Work out the finished part from the listing and answer in its coordinate system (mm). A direction names the side the tool comes from. Round coordinates to 2 decimals unless told otherwise and drop trailing zeros. Loops run counter-clockwise (first coordinate to the right, second up) from the corner with the lowest first, then second, coordinate; pieces in that order, holes last. Notation, with made-up numbers: (48.5, 79) -> (63.5, 79) arc R25 cw to (63.5, 97) -> close; hole circle Ø8 at (-4, 88.25). An arc over 180 degrees is marked (long way). Use CSV: the item, a comma, the result in double quotes. Start each with the question number.
from build123d import *

# Parameters (mm, degrees)
BOSS_EXTRUDE1_DEPTH = 76.2
CUT_EXTRUDE1_DEPTH  = 105.116765701
SKETCH3_R           = 1.5875
CUT_EXTRUDE2_DEPTH  = 105.116765701


with BuildPart() as part:
    # Sketch1 → Boss-Extrude1 (new body)
    with BuildSketch(Plane(origin=(0, 0, 0), x_dir=(1, 0, 0), z_dir=(0, 1, 0))):
        Polygon((0, 0), (0, 1.27), (49.53, 1.27), (49.53, 50.8), (50.8, 50.8), (50.8, 0), align=None)
    extrude(amount=BOSS_EXTRUDE1_DEPTH)

    # Sketch2 → Cut-Extrude1 (cut, through all)
    with BuildSketch(Plane.ZY.offset(-49.53)):
        with BuildLine():
            ThreePointArc((-9.908, 58.446006351), (-9.856223305, 58.052723305), (-10.249506351, 58.1045))
            ThreePointArc((-10.249506351, 58.1045), (-10.341012702, 58.196006351), (-10.466012702, 58.2295))
            Line((-10.466012702, 58.2295), (-40.333987298, 58.2295))
            ThreePointArc((-40.333987298, 58.2295), (-40.458987298, 58.196006351), (-40.550493649, 58.1045))
            ThreePointArc((-40.550493649, 58.1045), (-40.943776695, 58.052723305), (-40.892, 58.446006351))
            ThreePointArc((-40.892, 58.446006351), (-40.800493649, 58.537512702), (-40.767, 58.662512702))
            Line((-40.767, 58.662512702), (-40.767, 68.337487298))
            ThreePointArc((-40.767, 68.337487298), (-40.800493649, 68.462487298), (-40.892, 68.553993649))
            ThreePointArc((-40.892, 68.553993649), (-40.943776695, 68.947276695), (-40.550493649, 68.8955))
            ThreePointArc((-40.550493649, 68.8955), (-40.458987298, 68.803993649), (-40.333987298, 68.7705))
            Line((-40.333987298, 68.7705), (-10.466012702, 68.7705))
            ThreePointArc((-10.466012702, 68.7705), (-10.341012702, 68.803993649), (-10.249506351, 68.8955))
            ThreePointArc((-10.249506351, 68.8955), (-9.856223305, 68.947276695), (-9.908, 68.553993649))
            ThreePointArc((-9.908, 68.553993649), (-9.999506351, 68.462487298), (-10.033, 68.337487298))
            Line((-10.033, 68.337487298), (-10.033, 58.662512702))
            ThreePointArc((-10.033, 58.662512702), (-9.999506351, 58.537512702), (-9.908, 58.446006351))
        make_face()
        with BuildLine():
            ThreePointArc((-9.908, 33.046006351), (-9.856223305, 32.652723305), (-10.249506351, 32.7045))
            ThreePointArc((-10.249506351, 32.7045), (-10.341012702, 32.796006351), (-10.466012702, 32.8295))
            Line((-10.466012702, 32.8295), (-40.333987298, 32.8295))
            ThreePointArc((-40.333987298, 32.8295), (-40.458987298, 32.796006351), (-40.550493649, 32.7045))
            ThreePointArc((-40.550493649, 32.7045), (-40.943776695, 32.652723305), (-40.892, 33.046006351))
            ThreePointArc((-40.892, 33.046006351), (-40.800493649, 33.137512702), (-40.767, 33.262512702))
            Line((-40.767, 33.262512702), (-40.767, 42.937487298))
            ThreePointArc((-40.767, 42.937487298), (-40.800493649, 43.062487298), (-40.892, 43.153993649))
            ThreePointArc((-40.892, 43.153993649), (-40.943776695, 43.547276695), (-40.550493649, 43.4955))
            ThreePointArc((-40.550493649, 43.4955), (-40.458987298, 43.403993649), (-40.333987298, 43.3705))
            Line((-40.333987298, 43.3705), (-10.466012702, 43.3705))
            ThreePointArc((-10.466012702, 43.3705), (-10.341012702, 43.403993649), (-10.249506351, 43.4955))
            ThreePointArc((-10.249506351, 43.4955), (-9.856223305, 43.547276695), (-9.908, 43.153993649))
            ThreePointArc((-9.908, 43.153993649), (-9.999506351, 43.062487298), (-10.033, 42.937487298))
            Line((-10.033, 42.937487298), (-10.033, 33.262512702))
            ThreePointArc((-10.033, 33.262512702), (-9.999506351, 33.137512702), (-9.908, 33.046006351))
        make_face()
        with BuildLine():
            ThreePointArc((-9.908, 7.646006351), (-9.856223305, 7.252723305), (-10.249506351, 7.3045))
            ThreePointArc((-10.249506351, 7.3045), (-10.341012702, 7.396006351), (-10.466012702, 7.4295))
            Line((-10.466012702, 7.4295), (-40.333987298, 7.4295))
            ThreePointArc((-40.333987298, 7.4295), (-40.458987298, 7.396006351), (-40.550493649, 7.3045))
            ThreePointArc((-40.550493649, 7.3045), (-40.943776695, 7.252723305), (-40.892, 7.646006351))
            ThreePointArc((-40.892, 7.646006351), (-40.800493649, 7.737512702), (-40.767, 7.862512702))
            Line((-40.767, 7.862512702), (-40.767, 17.537487298))
            ThreePointArc((-40.767, 17.537487298), (-40.800493649, 17.662487298), (-40.892, 17.753993649))
            ThreePointArc((-40.892, 17.753993649), (-40.943776695, 18.147276695), (-40.550493649, 18.0955))
            ThreePointArc((-40.550493649, 18.0955), (-40.458987298, 18.003993649), (-40.333987298, 17.9705))
            Line((-40.333987298, 17.9705), (-10.466012702, 17.9705))
            ThreePointArc((-10.466012702, 17.9705), (-10.341012702, 18.003993649), (-10.249506351, 18.0955))
            ThreePointArc((-10.249506351, 18.0955), (-9.856223305, 18.147276695), (-9.908, 17.753993649))
            ThreePointArc((-9.908, 17.753993649), (-9.999506351, 17.662487298), (-10.033, 17.537487298))
            Line((-10.033, 17.537487298), (-10.033, 7.862512702))
            ThreePointArc((-10.033, 7.862512702), (-9.999506351, 7.737512702), (-9.908, 7.646006351))
        make_face()
    extrude(amount=-CUT_EXTRUDE1_DEPTH, mode=Mode.SUBTRACT)

    # Sketch3 → Cut-Extrude2 (cut, through all)
    with BuildSketch(Plane(origin=(0, 0, -1.27), x_dir=(-1, 0, 0), z_dir=(0, 0, -1))):
        with Locations((-6.35, 69.85)):
            Circle(SKETCH3_R)
        with Locations((-6.35, 6.35)):
            Circle(SKETCH3_R)
        with Locations((-43.18, 6.35)):
            Circle(SKETCH3_R)
        with Locations((-43.18, 69.85)):
            Circle(SKETCH3_R)
    extrude(amount=-CUT_EXTRUDE2_DEPTH, mode=Mode.SUBTRACT)


solid = part.part
Q1. Section B-B, the plane z = -15.5 is taken. Write down the section's boundary in (x, y), and give its area (3 significant figures).
Q2. Straight lines are drawn through the part: line 1 (Y direction, x = 6.35, z = -0.4); line 2 (X direction, y = 69.85, z = -0.45); line 3 (Z direction, x = 44.5, y = 47). For each, find the intervals that lie inside material, in ascending order. Write a range as from..to.
Q3. Section A-A, the plane y = 66 is taken. Write down the section's boundary in (x, z).
Q4. For a pull along X with two mould halves and no side action, classify faces 1 (the flat face through (50.8, 29, -26)), 2 (the cylindrical face through (44.766, 69.92, -0.644)), 3 (the flat face through (24, 38, -1.27)), 4 (the cylindrical face through (44.766, 6.42, -0.644)) as pulls with the +X half, pulls with the -X half, needs draft (parallel to the pull), parting line crosses it, or undercut.
Q5. This flat-tipped pin is pushed along its axis until it touches: pin 1 (3 mm diameter, centred on x = 15, y = 39, fed in from -Z). Where does it stop, or does it pass through?
Q6. Which of the six approach directions +Z, -Z, +X, -X, +Y, -Y give full straight-line access (tool end or side, diameter ignored) to faces 5 (the flat face through (49.53, 29, -26)), 6 (the flat face through (37, 0, -1))?
Q7. Section D-D, the plane y = 50 is taken. Write down the section's boundary in (x, z).
Q8. Section C-C, the plane x = 6.35 is taken. Write down the section's boundary in (y, z).
Report:
1,outline,"(49.53, 0) -> (50.8, 0) -> (50.8, 7.43) -> (49.53, 7.43) -> close; (49.53, 17.97) -> (50.8, 17.97) -> (50.8, 32.83) -> (49.53, 32.83) -> close; (49.53, 43.37) -> (50.8, 43.37) -> (50.8, 58.23) -> (49.53, 58.23) -> close; (49.53, 68.77) -> (50.8, 68.77) -> (50.8, 76.2) -> (49.53, 76.2) -> close"
1,area,"56.6 mm²"
2,line 1,"y = 0..4.76, 7.94..68.26, 71.44..76.2"
2,line 2,"x = 0..4.76, 7.94..41.59, 44.77..50.8"
2,line 3,"z = -1.27..0"
3,outline,"(0, -1.27) -> (49.53, -1.27) -> (49.53, -10.03) -> (50.8, -10.03) -> (50.8, 0) -> (0, 0) -> close; (49.53, -50.8) -> (50.8, -50.8) -> (50.8, -40.77) -> (49.53, -40.77) -> close"
4,face 1,"pulls with the +X half"
4,face 2,"undercut"
4,face 3,"needs draft"
4,face 4,"undercut"
5,pin 1,"stops at z = -1.27"
6,face 5,"-Z, -X, +Y, -Y"
6,face 6,"+Z, -Z, +X, -X, -Y"
7,outline,"(0, -1.27) -> (49.53, -1.27) -> (49.53, -50.8) -> (50.8, -50.8) -> (50.8, 0) -> (0, 0) -> close"
8,outline,"(0, -1.27) -> (4.76, -1.27) -> (4.76, 0) -> (0, 0) -> close; (7.94, -1.27) -> (68.26, -1.27) -> (68.26, 0) -> (7.94, 0) -> close; (71.44, -1.27) -> (76.2, -1.27) -> (76.2, 0) -> (71.44, 0) -> close"
